Verification items for the finished model (mm, model axes). Face numbers are marked on the shaded views. A direction names the side the tool comes from. Round coordinates to 2 decimals unless told otherwise and drop trailing zeros. One line per question, with ' | ' between items. Start each with the question number.
Q1. Gauge pin test, flat ends, axial feed: pin 1 (0.8 mm diameter, centred on x = 1, y = 2.5, fed in from +Z); pin 2 (2 mm diameter, centred on y = 2, z = -2, fed in from -X). Record the tip position at first contact, or that the pin passes through.
Q2. Release check for a two-part mould opening along Z. For the marked faces 3 and 4 record: released by +Z, released by -Z, zero draft, split by the parting line, or undercut.
Q3. Thickness scan on line 1 along Z through (x, y) = (-1.25, 3.2); line 2 along Y through (x, z) = (0.25, 0); line 3 along Z through (x, y) = (0.5, 2.05). Record the ranges inside material, lowest first. Write a range as from..to.
Q4. Tool access check on the marked faces 1 and 2. Record the directions out of +Z, -Z, +X, -X, +Y, -Y that give a thin tool (end or side, any length) a straight path to the whole face; none if there is none.
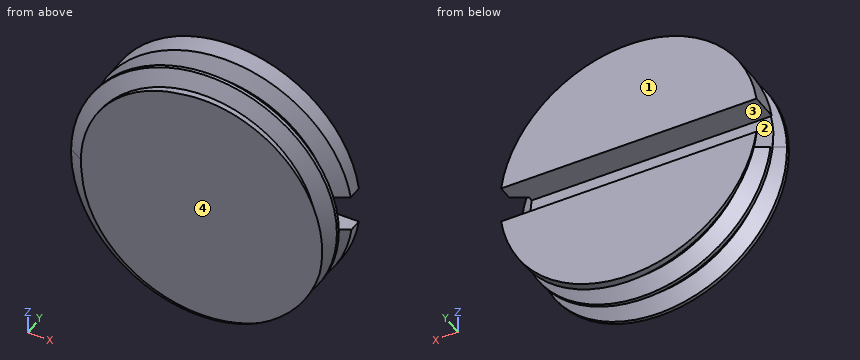
from build123d import *

# Parameters (mm, degrees)
SKETCH_1_R               = 7
EXTRUDE_1_DEPTH          = 3.5
THREAD_1_PITCH           = 1.5
CUT_EXTRUDE_1_DEPTH      = 11.5000004
CUT_EXTRUDE_1_DEPTH_BACK = 11.5000004
SKETCH_4_W               = 2
SKETCH_4_H               = 1.5


with BuildPart() as part:
    # Sketch 1 → Бобышка-Вытянуть1 (new body)
    with BuildSketch(Plane(origin=(0, 0, 0), x_dir=(1, 0, 0), z_dir=(0, 1, 0))):
        with Locations(Location((0, 0, 0), (0, 0, 270))):
            Circle(SKETCH_1_R)
    extrude(amount=EXTRUDE_1_DEPTH)

    # Резьба1: the profile of Sketch 1 2 profile screwed along a right-hand helix of 2.333333 turns, 8 arcs to a turn; built about Z, then put on its axis
    thread_1_z = Axis((0, 0, 0), (0, 0, 1))
    thread_1_corners = [(7.0003, 0, -0.000173205), (7.0003, 0, 1.312673201), (6.188101188, 0, 0.843749998), (6.188101188, 0, 0.468749998)]
    with BuildLine(mode=Mode.PRIVATE) as thread_1_profile:
        Line(thread_1_corners[0], thread_1_corners[1])
        Line(thread_1_corners[1], thread_1_corners[2])
        Line(thread_1_corners[2], thread_1_corners[3])
        Line(thread_1_corners[3], thread_1_corners[0])
    thread_1_cap = Face(thread_1_profile.wire())
    thread_1_turn_angles = [0, 22.5, 45, 67.5, 90, 112.5, 135, 157.5, 180, 202.5, 225, 247.5, 270, 292.5, 315, 337.5, 360]
    thread_1_turn_weights = [1, 0.9238795325112867, 1, 0.9238795325112867, 1, 0.9238795325112867, 1, 0.9238795325112867, 1, 0.9238795325112867, 1, 0.9238795325112867, 1, 0.9238795325112867, 1, 0.9238795325112867, 1]
    thread_1_turn_rails = [Edge.make_bspline([Vector(p[0], p[1], 0).rotate(thread_1_z, thread_1_turn_angles[k]) / thread_1_turn_weights[k] + Vector(0, 0, p[2] + THREAD_1_PITCH * thread_1_turn_angles[k] / 360) for k in range(17)], [0, 0, 0, 1, 1, 2, 2, 3, 3, 4, 4, 5, 5, 6, 6, 7, 7, 8, 8, 8], 2, thread_1_turn_weights) for p in thread_1_corners]
    thread_1_turn_sides = [Face.make_surface_from_curves(thread_1_turn_rails[p[0]], thread_1_turn_rails[p[1]]) for p in [(0, 1), (1, 2), (2, 3), (3, 0)]]
    thread_1_last_angles = [720, 742.5, 765, 787.5, 810, 825, 840]
    thread_1_last_weights = [1, 0.9238795325112867, 1, 0.9238795325112867, 1, 0.9659258262890685, 1]
    thread_1_last_rails = [Edge.make_bspline([Vector(p[0], p[1], 0).rotate(thread_1_z, thread_1_last_angles[k]) / thread_1_last_weights[k] + Vector(0, 0, p[2] + THREAD_1_PITCH * thread_1_last_angles[k] / 360) for k in range(7)], [0, 0, 0, 1, 1, 2, 2, 3, 3, 3], 2, thread_1_last_weights) for p in thread_1_corners]
    thread_1_last_sides = [Face.make_surface_from_curves(thread_1_last_rails[p[0]], thread_1_last_rails[p[1]]) for p in [(0, 1), (1, 2), (2, 3), (3, 0)]]
    thread_1 = Plane(origin=(0, 3.5, 0), x_dir=(-1, 0, 0), z_dir=(0, -1, 0)) * Solid(Shell([*[p.moved(Location((0, 0, THREAD_1_PITCH * i))) for i in range(2) for p in thread_1_turn_sides], *thread_1_last_sides, thread_1_cap, thread_1_cap.rotate(thread_1_z, 840).moved(Location((0, 0, THREAD_1_PITCH * 840 / 360)))]))
    add(thread_1, mode=Mode.SUBTRACT)

    # Эскиз4 → Вырез-Вытянуть1 (cut, two sides: drawn at the far end of the back side and taken through both)
    with BuildSketch(Plane(origin=(0, 0, 0), x_dir=(0, 0, -1), z_dir=(1, 0, 0)).offset(-CUT_EXTRUDE_1_DEPTH_BACK)):
        with Locations((0, 2.75)):
            Rectangle(SKETCH_4_W, SKETCH_4_H)
    extrude(amount=CUT_EXTRUDE_1_DEPTH + CUT_EXTRUDE_1_DEPTH_BACK, mode=Mode.SUBTRACT)


solid = part.part
Determined:
1) pin 1: stops at z = 6.97 | pin 2: stops at x = -6.93
2) face 3: undercut | face 4: zero draft
3) line 1: z = -6.89..-1, 1..6.89 | line 2: y = 0..2 | line 3: z = -6.54..-1, 1..6.39
4) face 1: +Z, -Z, +X, -X, +Y | face 2: +X, -X, +Y
